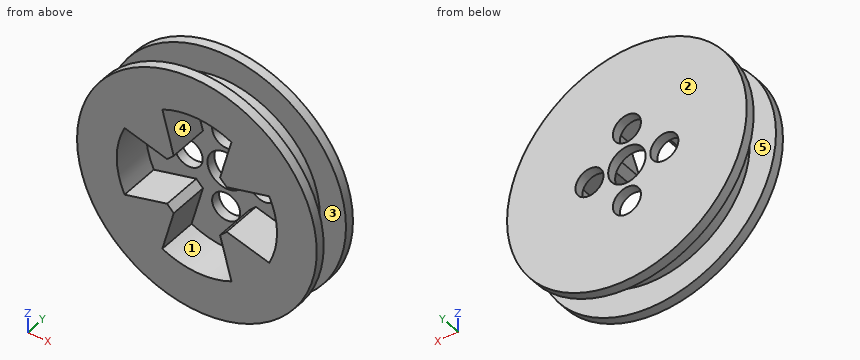
```python
from build123d import *

# Parameters (mm, degrees)
SKETCH1_R           = 20.32
SKETCH1_R_2         = 3.175
SKETCH1_R_3         = 2.38125
BOSS_EXTRUDE1_DEPTH = 1.5875
SKETCH2_R           = 15.875
SKETCH2_R_2         = 13.589
BOSS_EXTRUDE2_DEPTH = 5.08
SKETCH3_R           = 20.32
SKETCH3_R_2         = 13.589
BOSS_EXTRUDE3_DEPTH = 1.5875
BOSS_EXTRUDE4_DEPTH = 6.6675


with BuildPart() as part:
    # Sketch1 → Boss-Extrude1 (new body)
    with BuildSketch(Plane.XZ.offset(4.640864108)):
        with Locations((64.802565284, 12.446906686)):
            Circle(SKETCH1_R)
        with Locations((64.802565284, 12.446906686)):
            Circle(SKETCH1_R_2, mode=Mode.SUBTRACT)
        with Locations((58.452565284, 12.446906686)):
            Circle(SKETCH1_R_3, mode=Mode.SUBTRACT)
        with Locations((71.152565284, 12.446906686)):
            Circle(SKETCH1_R_3, mode=Mode.SUBTRACT)
        with Locations((64.802565284, 18.796906686)):
            Circle(SKETCH1_R_3, mode=Mode.SUBTRACT)
        with Locations((64.802565284, 6.096906686)):
            Circle(SKETCH1_R_3, mode=Mode.SUBTRACT)
    extrude(amount=BOSS_EXTRUDE1_DEPTH)

    # Sketch2 → Boss-Extrude2 (add)
    with BuildSketch(Plane.XZ.offset(6.228364108)):
        with Locations((64.802565284, 12.446906686)):
            Circle(SKETCH2_R)
        with Locations((64.802565284, 12.446906686)):
            Circle(SKETCH2_R_2, mode=Mode.SUBTRACT)
    extrude(amount=BOSS_EXTRUDE2_DEPTH)

    # Sketch3 → Boss-Extrude3 (add)
    with BuildSketch(Plane.XZ.offset(11.308364108)):
        with Locations((64.802565284, 12.446906686)):
            Circle(SKETCH3_R)
        with Locations((64.802565284, 12.446906686)):
            Circle(SKETCH3_R_2, mode=Mode.SUBTRACT)
    extrude(amount=BOSS_EXTRUDE3_DEPTH)

    # Sketch4 → Boss-Extrude4 (add)
    with BuildSketch(Plane.XZ.offset(6.228364108)):
        with BuildLine():
            Line((52.542239657, 18.307396129), (59.751171216, 16.375768739))
            Line((59.751171216, 16.375768739), (60.873703231, 17.498300754))
            Line((60.873703231, 17.498300754), (58.942075841, 24.707232314))
            ThreePointArc((58.942075841, 24.707232314), (55.193691235, 22.055780736), (52.542239657, 18.307396129))
        make_face()
        with BuildLine():
            Line((70.663054727, 24.707232314), (68.731427337, 17.498300754))
            Line((68.731427337, 17.498300754), (69.853959352, 16.375768739))
            Line((69.853959352, 16.375768739), (77.062890912, 18.307396129))
            ThreePointArc((77.062890912, 18.307396129), (74.411439334, 22.055780736), (70.663054727, 24.707232314))
        make_face()
        with BuildLine():
            Line((77.062890912, 6.586417243), (69.853959352, 8.518044633))
            Line((69.853959352, 8.518044633), (68.731427337, 7.395512618))
            Line((68.731427337, 7.395512618), (70.663054727, 0.186581059))
            ThreePointArc((70.663054727, 0.186581059), (74.411439334, 2.838032636), (77.062890912, 6.586417243))
        make_face()
        with BuildLine():
            Line((58.942075841, 0.186581059), (60.873703231, 7.395512618))
            Line((60.873703231, 7.395512618), (59.751171216, 8.518044633))
            Line((59.751171216, 8.518044633), (52.542239657, 6.586417243))
            ThreePointArc((52.542239657, 6.586417243), (55.193691235, 2.838032636), (58.942075841, 0.186581059))
        make_face()
    extrude(amount=BOSS_EXTRUDE4_DEPTH)


solid = part.part
```
The model under review builds one solid part; all positions refer to its coordinate system, in mm. Face numbers are marked on the shaded views. A direction names the side the tool comes from. Give positions to 0.01 mm unless a question says otherwise; leave off trailing zeros. Loops run counter-clockwise (first coordinate to the right, second up) from the corner with the lowest first, then second, coordinate; pieces in that order, holes last. Notation, with made-up numbers: (80, 28) -> (86, 28) arc R15 ccw to (86, 45) -> close; hole circle Ø7 at (68.5, 20.25). An arc over 180 degrees is marked (long way). Use CSV: the item, a comma, the result in double quotes.
1. Consider section B-B, the plane x = 65.5. Write out the cut boundary in (y, z).
Result:
outline,"(-12.9, -7.86) -> (-11.31, -7.86) -> (-11.31, -3.41) -> (-6.23, -3.41) -> (-6.23, -7.86) -> (-4.64, -7.86) -> (-4.64, 3.82) -> (-6.23, 3.82) -> (-6.23, -1.12) -> (-12.9, -1.12) -> close; (-12.9, 26.02) -> (-6.23, 26.02) -> (-6.23, 21.07) -> (-4.64, 21.07) -> (-4.64, 32.75) -> (-6.23, 32.75) -> (-6.23, 28.31) -> (-11.31, 28.31) -> (-11.31, 32.75) -> (-12.9, 32.75) -> close; (-6.23, 8.37) -> (-4.64, 8.37) -> (-4.64, 9.35) -> (-6.23, 9.35) -> close; (-6.23, 15.54) -> (-4.64, 15.54) -> (-4.64, 16.52) -> (-6.23, 16.52) -> close"
2. For P1, Ø1.5, axis at y = -10, z = 0, coming from the +X side; P2, Ø2, axis at y = -6.5, z = 16, coming from the -X side; P3, Ø1, axis at x = 54.5, y = -10, coming from the -Z side, all flat-tipped, find the tip position at first contact; note any pin that passes through.
Result:
P1,"stops at x = 75.54"
P2,"stops at x = 44.65"
P3,"stops at z = -0.04"
3. To check wall thickness, follow probe 1 along Y at (x, z) = (53, -2); probe 2 along Y at (x, z) = (69, 20); probe 3 along X at (y, z) = (-10, 21.5). State the ranges of each line that lie inside material, in increasing order. Write a range as from..to.
Result:
probe 1,"y = -12.9..-11.31, -6.23..-4.64"
probe 2,"y = -6.23..-4.64"
probe 3,"x = 51.76..59.8, 69.8..77.84"
4. Consider section C-C, the plane x = 82. Write out the cut boundary in (y, z).
Result:
outline,"(-12.9, 1.62) -> (-11.31, 1.62) -> (-11.31, 23.27) -> (-12.9, 23.27) -> close; (-6.23, 1.62) -> (-4.64, 1.62) -> (-4.64, 23.27) -> (-6.23, 23.27) -> close"
5. Machinability: for the marked faces 1, 2 and 3, which of the approach directions +Z, -Z, +X, -X, +Y, -Y give a long, thin tool a straight path to every point of the face, cutting with its end or side? Answer none if there is none.
Result:
face 1,"-Y"
face 2,"+Z, -Z, +X, -X, +Y"
face 3,"none"
6. Consider section D-D, the plane z = -2. Write out the cut boundary in (x, y).
Result:
outline,"(50.51, -12.9) -> (79.09, -12.9) -> (79.09, -11.31) -> (71.38, -11.31) -> (71.38, -6.23) -> (79.09, -6.23) -> (79.09, -4.64) -> (50.51, -4.64) -> (50.51, -6.23) -> (58.22, -6.23) -> (58.22, -11.31) -> (50.51, -11.31) -> close"
7. Consider section A-A, the plane y = -10. Write out the cut boundary in (x, z) (3 decimals).
Result:
outline,"circle Ø31.75 at (64.803, 12.447); hole (52.542, 6.586) -> (59.751, 8.518) -> (60.874, 7.396) -> (58.942, 0.187) arc R13.589 ccw to (70.663, 0.187) -> (68.731, 7.396) -> (69.854, 8.518) -> (77.063, 6.586) arc R13.589 ccw to (77.063, 18.307) -> (69.854, 16.376) -> (68.731, 17.498) -> (70.663, 24.707) arc R13.589 ccw to (58.942, 24.707) -> (60.874, 17.498) -> (59.751, 16.376) -> (52.542, 18.307) arc R13.589 ccw to start"
8. The part is to be moulded in two halves that separate along Z. For the marked faces 4 and 5, say which applies: +Z half, -Z half, draft (parallel to the pull), parting line (faces both ways), or undercut.
Result:
face 4,"undercut"
face 5,"draft"
